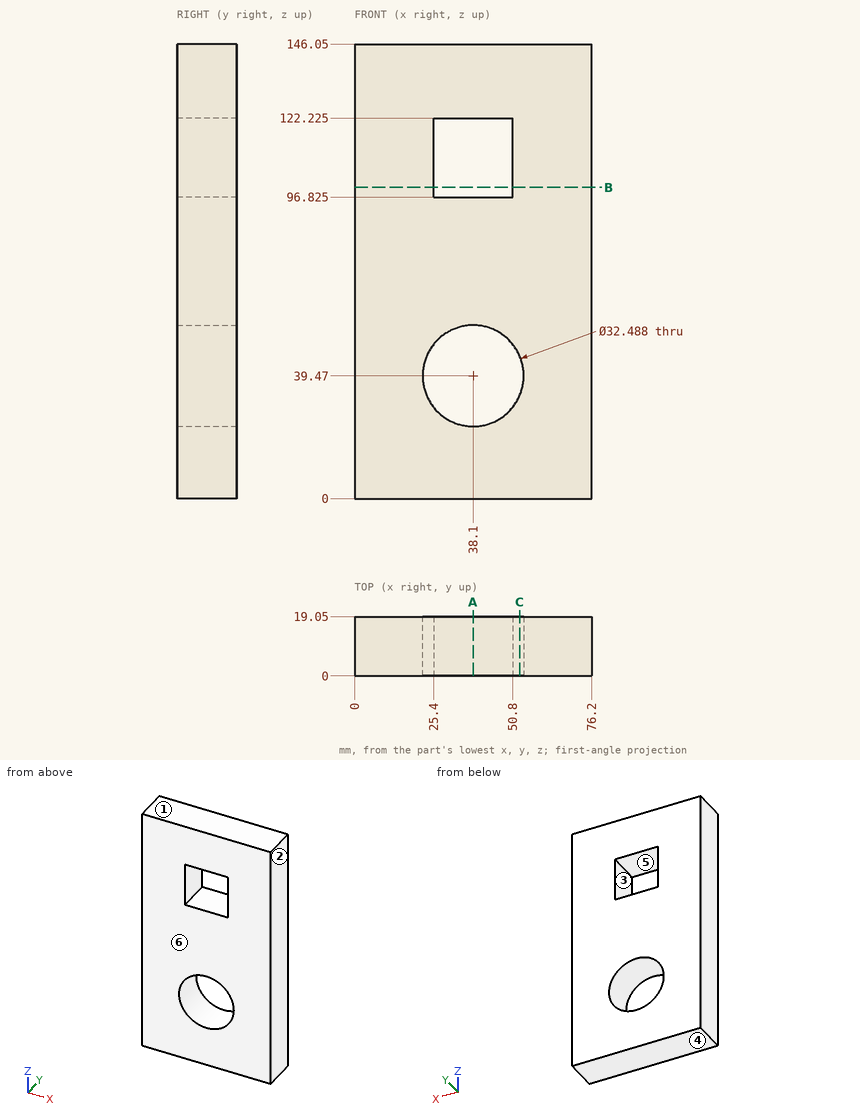
The drawing under review shows one solid part. Ordinate dimensions are in mm from its lowest x, y, z. A direction names the side the tool comes from. Coordinates: 2 decimals unless noted, no trailing zeros. Loops run counter-clockwise (first coordinate to the right, second up) from the corner with the lowest first, then second, coordinate; pieces in that order, holes last. Notation, with made-up numbers: (-8.5, 37) - (30.5, 37) arc R32 ccw to (30.5, 66) - close; hole circle Ø5 at (36.25, 71.25). An arc over 180 degrees is marked (long way). Return JSON: item names as keys, results as strings.
Item 1: For the marked faces 5 and 6, list the 3-axis set-ups (+Z, -Z, +X, -X, +Y, -Y) from which the entire face can be reached by the end or side of a thin tool; tool diameter is ignored.
Determined:
{"face 5": "+Y, -Y", "face 6": "+Z, -Z, +X, -X, -Y"}
Item 2: Take a section at C-C (x = 53). Give the boundary of the cut face in (y, z).
Determined:
{"outline": "(0, 0) - (19.05, 0) - (19.05, 33) - (0, 33) - close; (0, 45.94) - (19.05, 45.94) - (19.05, 146.05) - (0, 146.05) - close"}
Item 3: For line 1 (X direction, y = 7, z = 101); line 2 (X direction, y = 14.5, z = 42), list the stretches that pass through material, from the lowest coordinate up.
Determined:
{"line 1": "x = 0 to 25.4, 50.8 to 76.2", "line 2": "x = 0 to 22.05, 54.15 to 76.2"}
Item 4: Mouldability with a two-part tool opening along Z and no side actions: class the marked faces 1, 2, 3 and 4 as pulls with the +Z half, pulls with the -Z half, needs draft (parallel to the pull), parting line crosses it, or undercut.
Determined:
{"face 1": "pulls with the +Z half", "face 2": "needs draft", "face 3": "undercut", "face 4": "pulls with the -Z half"}
Item 5: Take a section at A-A (x = 38.1). State how many separate pieces and enclosed holes the cut face has, then the cut area to 3 significant figures.
Determined:
{"separate pieces": "3", "enclosed holes": "0", "area": "1,680 mm2"}
Item 6: Take a section at B-B (z = 100). Give the boundary of the cut face in (x, y), then the cut area to 3 significant figures.
Determined:
{"outline": "(0, 0) - (25.4, 0) - (25.4, 19.05) - (0, 19.05) - close; (50.8, 0) - (76.2, 0) - (76.2, 19.05) - (50.8, 19.05) - close", "area": "968 mm2"}
